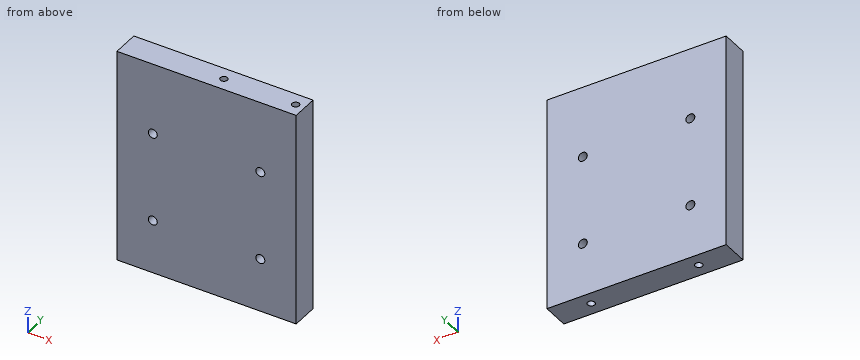
```python
from build123d import *

# Parameters (mm, degrees)
F0_W     = 127
F0_H     = 152.4
F0_R     = 3.175
F1_DEPTH = 19.05
F3_D     = 5.1054
F3_DEPTH = 25.4
F3_TIP   = 1.5338169022
F5_D     = 5.1054
F5_DEPTH = 25.4
F5_TIP   = 1.5338169022
F6_D     = 5.1054
F6_DEPTH = 25.4
F6_TIP   = 1.5338169022


with BuildPart() as f1:
    # F0 (on Front) → F1 (new body)
    with BuildSketch(Plane.XZ):
        with Locations((-63.5, 76.2)):
            Rectangle(F0_W, F0_H)
        with Locations((-101.6, 38.1)):
            Circle(F0_R, mode=Mode.SUBTRACT)
        with Locations((-25.4, 38.1)):
            Circle(F0_R, mode=Mode.SUBTRACT)
        with Locations((-101.6, 101.6)):
            Circle(F0_R, mode=Mode.SUBTRACT)
        with Locations((-25.4, 101.6)):
            Circle(F0_R, mode=Mode.SUBTRACT)
    extrude(amount=F1_DEPTH)

    # F3
    with Locations(Plane(origin=(0, 0, 0), x_dir=(1, 0, 0), z_dir=(0, 0, -1))):
        with Locations((-101.6, 9.525), (-25.4, 9.525)):
            Hole(F3_D / 2, depth=F3_DEPTH)
            with Locations((0, 0, -(F3_DEPTH + F3_TIP / 2))):  # 118° drill point
                Cone(0, F3_D / 2, F3_TIP, mode=Mode.SUBTRACT)

    # F5
    with Locations(Plane.XY.offset(152.4)):
        with Locations((-57.15, -9.525)):
            Hole(F5_D / 2, depth=F5_DEPTH)
            with Locations((0, 0, -(F5_DEPTH + F5_TIP / 2))):  # 118° drill point
                Cone(0, F5_D / 2, F5_TIP, mode=Mode.SUBTRACT)

    # F6
    with Locations(Plane.XY.offset(152.4)):
        with Locations((-6.35, -9.525)):
            Hole(F6_D / 2, depth=F6_DEPTH)
            with Locations((0, 0, -(F6_DEPTH + F6_TIP / 2))):  # 118° drill point
                Cone(0, F6_D / 2, F6_TIP, mode=Mode.SUBTRACT)


solid = f1.part
```
Read the model definition and answer for the solid it produces. Units are mm, in the model's axes. Give positions to 0.01 mm unless a question says otherwise; leave off trailing zeros. Order: outer loops, then holes, each group sorted by start corner. A loop starts at its lowest first (then second) coordinate and runs counter-clockwise, first axis right, second up.
(1) Given pin 1 (4 mm diameter, centred on x = -6.35, y = -9.525, fed in from +Z); pin 2 (3 mm diameter, centred on x = -79, z = 26, fed in from +Y); pin 3 (4 mm diameter, centred on x = -101.6, z = 101.6, fed in from -Y); pin 4 (4 mm diameter, centred on x = -101.6, y = -9.525, fed in from -Z), each flat-ended and moving along its own axis, determine where each tip first touches the part or whether it passes through.
(2) Straight lines are drawn through the part: L1, parallel to Z at x = -101.5, y = -12.5; L2, parallel to X at y = -8.75, z = 131.5; L3, parallel to Y at x = -6.35, z = 142. For each, find the intervals that lie inside material, in ascending order.
(3) Find section A-A (z = 38.1). Give the vertices of the cut face in (x, y) (3 decimals), plus the area to 3 significant figures.
(4) Find section B-B (z = 16). Give the vertices of the cut face in (x, y) (3 decimals).
Result sheet:
1. pin 1: stops at z = 126.67
1. pin 2: stops at y = 0
1. pin 3: passes through
1. pin 4: stops at z = 25.73
2. L1: z = 0 to 34.93, 41.27 to 98.43, 104.77 to 152.4
2. L2: x = -127 to -59.58, -54.72 to -8.78, -3.92 to 0
2. L3: y = -19.05 to -12.08, -6.97 to 0
3. outline: (-127, -19.05) - (-104.775, -19.05) - (-104.775, 0) - (-127, 0) - close; (-98.425, -19.05) - (-28.575, -19.05) - (-28.575, 0) - (-98.425, 0) - close; (-22.225, -19.05) - (0, -19.05) - (0, 0) - (-22.225, 0) - close
3. area: 2,180 mm2
4. outline: (-127, -19.05) - (0, -19.05) - (0, 0) - (-127, 0) - close; hole circle Ø5.105 at (-101.6, -9.525); hole circle Ø5.105 at (-25.4, -9.525)
